The listing builds one solid part. Answer for the finished solid, in the listing's coordinates (mm). Face numbers are marked on the shaded views. A direction names the side the tool comes from. Round coordinates to 2 decimals unless told otherwise and drop trailing zeros. Write each loop counter-clockwise with the first axis right and the second up, starting at its lowest first coordinate (ties: lowest second). Pieces come first, ordered by that corner, then holes. Notation, with made-up numbers: (-15, 64) - (-7, 64) arc R25 ccw to (-7, 103) - close; hole circle Ø1 at (52, 68.25). An arc over 180 degrees is marked (long way). Return JSON: item names as keys, results as strings. Group by question number.
(1) Find the intervals of material crossed by line 1 along Z through (x, y) = (-19, 1.15); line 2 along Y through (x, z) = (-14, -1); line 3 along Z through (x, y) = (-2, 8.25), in increasing order. Write a range as [from, to].
(2) Section C-C, the plane x = 18 is taken. Write down the section's boundary in (y, z), then the cut area to 3 significant figures.
(3) Which of the six approach directions +Z, -Z, +X, -X, +Y, -Y give full straight-line access (tool end or side, diameter ignored) to the marked faces 1 and 2?
(4) Section B-B, the plane z = -0.35 is taken. Give the number of separate pieces and of enclosed holes in the cut face, then the cut area to 3 significant figures.
(5) Section A-A, the plane x = 11 is taken. Write down the section's boundary in (y, z).
(6) Each of these flat-tipped pins is pushed along its axis until it touches: pin 1 (2.5 mm diameter, centred on x = 11, z = 0, fed in from +Y); pin 2 (1.6 mm diameter, centred on x = 14.5, y = 1.5, fed in from +Z). Where does it stop, or does it pass through?
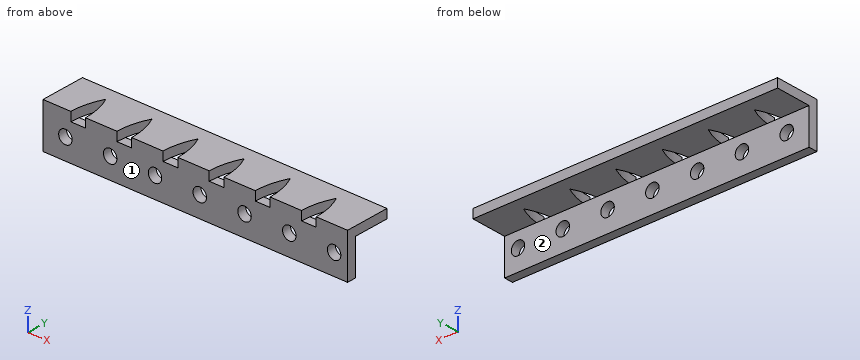
```python
from build123d import *

# Parameters (mm, degrees)
SKETCH1_W                      = 68
SKETCH1_H                      = 10
SKETCH1_R                      = 1.5025
BOSS_EXTRUDE1_DEPTH            = 10
CUT_EXTRUDE1_REACH             = 7
SKETCH2_W                      = 68
SKETCH2_H                      = 8
CUT_EXTRUDE1_DIRECTION_2_DEPTH = 3
CUT_EXTRUDE2_DEPTH             = 2


with BuildPart() as part:
    # Sketch1 → Boss-Extrude1 (new body)
    with BuildSketch(Plane(origin=(0, 0, 0), x_dir=(1, 0, 0), z_dir=(0, 1, 0))):
        Rectangle(SKETCH1_W, SKETCH1_H)
        with Locations((-29, 0.35)):
            Circle(SKETCH1_R, mode=Mode.SUBTRACT)
        with Locations((-19, 0.35)):
            Circle(SKETCH1_R, mode=Mode.SUBTRACT)
        with Locations((-9, 0.35)):
            Circle(SKETCH1_R, mode=Mode.SUBTRACT)
        with Locations((1, 0.35)):
            Circle(SKETCH1_R, mode=Mode.SUBTRACT)
        with Locations((11, 0.35)):
            Circle(SKETCH1_R, mode=Mode.SUBTRACT)
        with Locations((21, 0.35)):
            Circle(SKETCH1_R, mode=Mode.SUBTRACT)
        with Locations((31, 0.35)):
            Circle(SKETCH1_R, mode=Mode.SUBTRACT)
    extrude(amount=BOSS_EXTRUDE1_DEPTH)

    # Sketch2 → Cut-Extrude1 (cut, up to next)
    with BuildSketch(Plane.XY, mode=Mode.PRIVATE) as cut_extrude1_sk1:
        with Locations((0, 6)):
            Rectangle(SKETCH2_W, SKETCH2_H)
    cut_extrude1_tool1 = extrude(cut_extrude1_sk1.sketch, amount=-CUT_EXTRUDE1_REACH, mode=Mode.PRIVATE) & part.part
    add(cut_extrude1_tool1.solids().sort_by_distance((0, 6, 0))[0], mode=Mode.SUBTRACT)

    # Sketch2 → Cut-Extrude1 direction 2 (cut)
    with BuildSketch(Plane.XY):
        with Locations((0, 6)):
            Rectangle(SKETCH2_W, SKETCH2_H)
    extrude(amount=CUT_EXTRUDE1_DIRECTION_2_DEPTH, mode=Mode.SUBTRACT)

    # Sketch3 → Cut-Extrude2 (cut)
    with BuildSketch(Plane.XY.offset(5)):
        with BuildLine():
            Line((23.7, 0), (27, 0))
            add(Edge.make_bspline(
                [(25.35, 7), (26.975838532, 3.728518175), (27, 0)],
                knots=[0, 0, 0, 1, 1, 1], degree=2))
            add(Edge.make_bspline(
                [(25.35, 7), (23.724161468, 3.728518175), (23.7, 0)],
                knots=[0, 0, 0, 1, 1, 1], degree=2))
        make_face()
        with BuildLine():
            Line((13.4, 0), (16.7, 0))
            add(Edge.make_bspline(
                [(15.05, 7), (16.675838532, 3.728518175), (16.7, 0)],
                knots=[0, 0, 0, 1, 1, 1], degree=2))
            add(Edge.make_bspline(
                [(15.05, 7), (13.424161468, 3.728518175), (13.4, 0)],
                knots=[0, 0, 0, 1, 1, 1], degree=2))
        make_face()
        with BuildLine():
            Line((3.1, 0), (6.4, 0))
            add(Edge.make_bspline(
                [(4.75, 7), (6.375838532, 3.728518175), (6.4, 0)],
                knots=[0, 0, 0, 1, 1, 1], degree=2))
            add(Edge.make_bspline(
                [(4.75, 7), (3.124161468, 3.728518175), (3.1, 0)],
                knots=[0, 0, 0, 1, 1, 1], degree=2))
        make_face()
        with BuildLine():
            Line((-7.2, 0), (-3.9, 0))
            add(Edge.make_bspline(
                [(-5.55, 7), (-3.924161468, 3.728518175), (-3.9, 0)],
                knots=[0, 0, 0, 1, 1, 1], degree=2))
            add(Edge.make_bspline(
                [(-5.55, 7), (-7.175838532, 3.728518175), (-7.2, 0)],
                knots=[0, 0, 0, 1, 1, 1], degree=2))
        make_face()
        with BuildLine():
            Line((-17.5, 0), (-14.2, 0))
            add(Edge.make_bspline(
                [(-15.85, 7), (-14.224161468, 3.728518175), (-14.2, 0)],
                knots=[0, 0, 0, 1, 1, 1], degree=2))
            add(Edge.make_bspline(
                [(-15.85, 7), (-17.475838532, 3.728518175), (-17.5, 0)],
                knots=[0, 0, 0, 1, 1, 1], degree=2))
        make_face()
        with BuildLine():
            Line((-27.8, 0), (-24.5, 0))
            add(Edge.make_bspline(
                [(-26.15, 7), (-24.524161468, 3.728518175), (-24.5, 0)],
                knots=[0, 0, 0, 1, 1, 1], degree=2))
            add(Edge.make_bspline(
                [(-26.15, 7), (-27.775838532, 3.728518175), (-27.8, 0)],
                knots=[0, 0, 0, 1, 1, 1], degree=2))
        make_face()
    extrude(amount=-CUT_EXTRUDE2_DEPTH, mode=Mode.SUBTRACT)


solid = part.part
```
Working result:
{
 "1": {"line 1": "z = [-5, -1.85], [1.15, 5]", "line 2": "y = [0, 2]", "line 3": "z = [3, 5]"},
 "2": {"outline": "(0, -5) - (2, -5) - (2, 3) - (10, 3) - (10, 5) - (0, 5) - close", "area": "36.0 mm^2"},
 "3": {"face 1": "+Z, -Z, +X, -X, -Y", "face 2": "-Z, +X, -X, +Y"},
 "4": {"separate pieces": "8", "enclosed holes": "0", "area": "93.9 mm^2"},
 "5": {"outline": "(0, -5) - (2, -5) - (2, -1.85) - (0, -1.85) - close; (0, 1.15) - (2, 1.15) - (2, 3) - (10, 3) - (10, 5) - (0, 5) - close"},
 "6": {"pin 1": "stops at y = 2", "pin 2": "stops at z = 3"}
}
